```python
from build123d import *

# Parameters (mm, degrees)
F0_R     = 1.6
F0_R_2   = 1.25
F1_DEPTH = 3.175


# Not quite as in the source:
# - a length typed as a fraction of an inch, garbled in the dataset ("3 / 203.2 mm" for 3/8 in), is restored


with BuildPart() as f1:
    # F0 (on Front) → F1 (new body)
    with BuildSketch(Plane.XZ):
        with BuildLine():
            Line((61.44, 12.45), (-10.94, 12.45))
            ThreePointArc((-10.94, 12.45), (-13.6340768363, 11.3340768363), (-14.75, 8.64))
            Line((-14.75, 8.64), (-14.75, -33.74))
            ThreePointArc((-14.75, -33.74), (-13.6340768363, -36.4340768363), (-10.94, -37.55))
            Line((-10.94, -37.55), (61.44, -37.55))
            ThreePointArc((61.44, -37.55), (64.1340768363, -36.4340768363), (65.25, -33.74))
            Line((65.25, -33.74), (65.25, 8.64))
            ThreePointArc((65.25, 8.64), (64.1340768363, 11.3340768363), (61.44, 12.45))
        make_face()
        with Locations((-9.75, -32.55)):
            Circle(F0_R, mode=Mode.SUBTRACT)
        with Locations((0.25, -32.55)):
            Circle(F0_R, mode=Mode.SUBTRACT)
        with Locations((10.25, -32.55)):
            Circle(F0_R, mode=Mode.SUBTRACT)
        with Locations((20.25, -32.55)):
            Circle(F0_R, mode=Mode.SUBTRACT)
        with Locations((-9.75, -22.55)):
            Circle(F0_R, mode=Mode.SUBTRACT)
        with Locations((30.25, -32.55)):
            Circle(F0_R, mode=Mode.SUBTRACT)
        with Locations((40.25, -32.55)):
            Circle(F0_R, mode=Mode.SUBTRACT)
        with Locations((50.25, -32.55)):
            Circle(F0_R, mode=Mode.SUBTRACT)
        with Locations((60.25, -32.55)):
            Circle(F0_R, mode=Mode.SUBTRACT)
        with Locations((60.25, -22.55)):
            Circle(F0_R, mode=Mode.SUBTRACT)
        with Locations((-9.75, -12.55)):
            Circle(F0_R, mode=Mode.SUBTRACT)
        with Locations((1.75, -12.55)):
            Circle(F0_R_2, mode=Mode.SUBTRACT)
        with Locations((-9.75, -2.55)):
            Circle(F0_R, mode=Mode.SUBTRACT)
        with Locations((-9.75, 7.45)):
            Circle(F0_R, mode=Mode.SUBTRACT)
        with Locations((0.25, 7.45)):
            Circle(F0_R, mode=Mode.SUBTRACT)
        with Locations((10.25, 7.45)):
            Circle(F0_R, mode=Mode.SUBTRACT)
        with Locations((20.25, 7.45)):
            Circle(F0_R, mode=Mode.SUBTRACT)
        Polygon((26.75, -4.25), (36.75, -4.25), (36.75, 3.25), (55.5, 3.25), (55.5, -28.35), (-3.25, -28.35), (-3.25, -17.55), (4.25, -17.55), (4.25, -7.55), (-3.25, -7.55), (-3.25, 3.25), (26.75, 3.25), align=None, mode=Mode.SUBTRACT)
        with Locations((31.75, -1.75)):
            Circle(F0_R_2, mode=Mode.SUBTRACT)
        with Locations((60.25, -12.55)):
            Circle(F0_R, mode=Mode.SUBTRACT)
        with Locations((60.25, -2.55)):
            Circle(F0_R, mode=Mode.SUBTRACT)
        with Locations((30.25, 7.45)):
            Circle(F0_R, mode=Mode.SUBTRACT)
        with Locations((40.25, 7.45)):
            Circle(F0_R, mode=Mode.SUBTRACT)
        with Locations((50.25, 7.45)):
            Circle(F0_R, mode=Mode.SUBTRACT)
        with Locations((60.25, 7.45)):
            Circle(F0_R, mode=Mode.SUBTRACT)
    extrude(amount=F1_DEPTH)


solid = f1.part
```
Can you work these out from the model? Positions are in its coordinate system, mm. A direction names the side the tool comes from. Give positions to 0.01 mm unless a question says otherwise; leave off trailing zeros. Order: outer loops, then holes, each group sorted by start corner. A loop starts at its lowest first (then second) coordinate and runs counter-clockwise, first axis right, second up. Notation, with made-up numbers: M -31.75,82.5 L -11.75,82.5 A25 ccw -11.75,111.5 Z; hole C 35.25,-2.75 d10. An arc over 180 degrees is marked long. One line per item, written item: value.
1) On a 3-axis mill with a long thin cutter (end or side, diameter ignored), from which of +Z, -Z, +X, -X, +Y, -Y can I reach the whole of each face in a straight line? I mean faces 5 (the face through (64.164, -1.565, 11.304)), 6 (the face through (12, -2, 3.25)). Say none if no direction works.
Answer sheet:
face 5: +Z, +X, +Y, -Y
face 6: +Y, -Y
2) We'd pull the mould along X, two halves only. Please class faces 1 (the face through (50.99, -1.57, -33.97)), 2 (the face through (61.73, -1.57, -13.16)), 3 (the face through (26, -2, 12.45)), 4 (the face through (-13.664, -1.565, -36.404)): released by +X, released by -X, zero draft, split by the parting line, or undercut.
Answer sheet:
face 1: undercut
face 2: undercut
face 3: zero draft
face 4: released by -X
3) I want a section at B-B, the plane x = 10.25. List the corners of the cut face in (y, z) for me (3 decimals), plus the area to 3 significant figures.
Answer sheet:
outline: M -3.175,-37.55 L 0,-37.55 L 0,-34.15 L -3.175,-34.15 Z; M -3.175,-30.95 L 0,-30.95 L 0,-28.35 L -3.175,-28.35 Z; M -3.175,3.25 L 0,3.25 L 0,5.85 L -3.175,5.85 Z; M -3.175,9.05 L 0,9.05 L 0,12.45 L -3.175,12.45 Z
area: 38.1 mm^2
4) Please list where these lines run through material, in increasing order: line 1 along Z through (x, y) = (50, -2.35); line 2 along Z through (x, y) = (0.25, -1.5); line 3 along X through (y, z) = (-2.7, 2).
Answer sheet:
line 1: z = -37.55 to -34.13, -30.97 to -28.35, 3.25 to 5.87, 9.03 to 12.45
line 2: z = -37.55 to -34.15, -30.95 to -28.35, -17.55 to -7.55, 3.25 to 5.85, 9.05 to 12.45
line 3: x = -14.75 to -3.25, 26.75 to 36.75, 55.5 to 65.25
5) I want a section at C-C, the plane z = -6. List the corners of the cut face in (x, y) for me (3 decimals), plus the area to 3 significant figures.
Answer sheet:
outline: M -14.75,-3.175 L -3.25,-3.175 L -3.25,0 L -14.75,0 Z; M 55.5,-3.175 L 65.25,-3.175 L 65.25,0 L 55.5,0 Z
area: 67.5 mm^2
6) I want a section at D-D, the plane x = -9.75. List the corners of the cut face in (y, z) for me (3 decimals).
Answer sheet:
outline: M -3.175,-37.55 L 0,-37.55 L 0,-34.15 L -3.175,-34.15 Z; M -3.175,-30.95 L 0,-30.95 L 0,-24.15 L -3.175,-24.15 Z; M -3.175,-20.95 L 0,-20.95 L 0,-14.15 L -3.175,-14.15 Z; M -3.175,-10.95 L 0,-10.95 L 0,-4.15 L -3.175,-4.15 Z; M -3.175,-0.95 L 0,-0.95 L 0,5.85 L -3.175,5.85 Z; M -3.175,9.05 L 0,9.05 L 0,12.45 L -3.175,12.45 Z
7) I want a section at A-A, the plane z = -22.55. List the corners of the cut face in (x, y) for me (3 decimals).
Answer sheet:
outline: M -14.75,-3.175 L -11.35,-3.175 L -11.35,0 L -14.75,0 Z; M -8.15,-3.175 L -3.25,-3.175 L -3.25,0 L -8.15,0 Z; M 55.5,-3.175 L 58.65,-3.175 L 58.65,0 L 55.5,0 Z; M 61.85,-3.175 L 65.25,-3.175 L 65.25,0 L 61.85,0 Z
